Can you work these out from the model? Positions are in its coordinate system, mm. Coordinates: 2 decimals unless noted, no trailing zeros. Loops run counter-clockwise (first coordinate to the right, second up) from the corner with the lowest first, then second, coordinate; pieces in that order, holes last. Notation, with made-up numbers: M 86.5,-19.5 L 100.5,-19.5 A23 cw 100.5,1.5 Z; hole C 75,-29 d1. An arc over 180 degrees is marked long. Answer as a JSON object with one key per item and string values. Group by question number.
Item 1: Suppose I cut it at A-A (z = -2.5). Write out the boundary of the cut face in (x, y).
Item 2: I'm going to push flat-ended pins straight in: pin 1 Ø1.1 at (y, z) = (1.5, -24) entering from +X; pin 2 Ø1.5 at (x, z) = (1, 35.5) entering from -Y; pin 3 Ø0.7 at (y, z) = (1.5, -13) entering from -X; pin 4 Ø1.2 at (x, z) = (0, -3.5) entering from +Y. Where does each tip first touch, or does it pass through?
Item 3: Suppose I cut it at B-B (x = 0). Write out the boundary of the cut face in (y, z).
Item 4: Suppose I cut it at C-C (y = 1.6). Write out the boundary of the cut face in (x, z).
Item 5: If I drill on line 1 (Z direction, x = -0.05, y = 3.7); line 2 (Y direction, x = 1.05, z = -36); line 3 (X direction, y = 1.6, z = 16.5), over which ranges is the centre line in solid material (lowest first)?
```python
from build123d import *

# Parameters (mm, degrees)
SKETCH1_W           = 2.5
SKETCH1_H           = 105
BOSS_EXTRUDE1_DEPTH = 0.8
SKETCH2_W           = 1.9
SKETCH2_H           = 105
BOSS_EXTRUDE2_DEPTH = 1.4
SKETCH3_W           = 2.5
SKETCH3_H           = 105
BOSS_EXTRUDE3_DEPTH = 0.8
SKETCH4_R           = 0.65
BOSS_EXTRUDE4_DEPTH = 0.9


with BuildPart() as part:
    # Sketch1 → Boss-Extrude1 (new body)
    with BuildSketch(Plane(origin=(0, 0, 0), x_dir=(1, 0, 0), z_dir=(0, 1, 0))):
        Rectangle(SKETCH1_W, SKETCH1_H)
    extrude(amount=BOSS_EXTRUDE1_DEPTH)

    # Sketch2 → Boss-Extrude2 (add)
    with BuildSketch(Plane(origin=(0, 0.8, 0), x_dir=(1, 0, 0), z_dir=(0, 1, 0))):
        Rectangle(SKETCH2_W, SKETCH2_H)
    extrude(amount=BOSS_EXTRUDE2_DEPTH)

    # Sketch3 → Boss-Extrude3 (add)
    with BuildSketch(Plane(origin=(0, 2.2, 0), x_dir=(1, 0, 0), z_dir=(0, 1, 0))):
        Rectangle(SKETCH3_W, SKETCH3_H)
    extrude(amount=BOSS_EXTRUDE3_DEPTH)

    # Sketch4 → Boss-Extrude4 (add)
    with BuildSketch(Plane(origin=(0, 3, 0), x_dir=(1, 0, 0), z_dir=(0, 1, 0))):
        with Locations(Location((0, 18.75, 0), (0, 0, 270))):
            Circle(SKETCH4_R)
        with Locations(Location((0, -18.75, 0), (0, 0, 270))):
            Circle(SKETCH4_R)
        with Locations(Location((0, 48.75, 0), (0, 0, 270))):
            Circle(SKETCH4_R)
        with Locations(Location((0, -48.75, 0), (0, 0, 270))):
            Circle(SKETCH4_R)
    extrude(amount=BOSS_EXTRUDE4_DEPTH)


solid = part.part
```
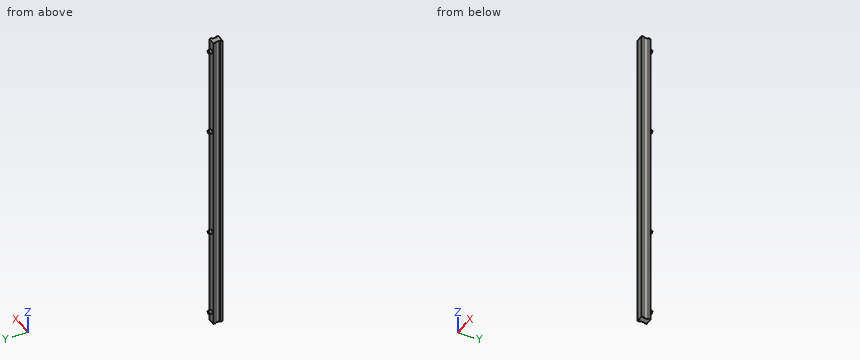
From the geometry:
{
 "1": {"outline": "M -1.25,0 L 1.25,0 L 1.25,0.8 L 0.95,0.8 L 0.95,2.2 L 1.25,2.2 L 1.25,3 L -1.25,3 L -1.25,2.2 L -0.95,2.2 L -0.95,0.8 L -1.25,0.8 Z"},
 "2": {"pin 1": "x = 0.95", "pin 2": "y = 0", "pin 3": "x = -0.95", "pin 4": "y = 3"},
 "3": {"outline": "M 0,-52.5 L 3,-52.5 L 3,-49.4 L 3.9,-49.4 L 3.9,-48.1 L 3,-48.1 L 3,-19.4 L 3.9,-19.4 L 3.9,-18.1 L 3,-18.1 L 3,18.1 L 3.9,18.1 L 3.9,19.4 L 3,19.4 L 3,48.1 L 3.9,48.1 L 3.9,49.4 L 3,49.4 L 3,52.5 L 0,52.5 Z"},
 "4": {"outline": "M -0.95,-52.5 L 0.95,-52.5 L 0.95,52.5 L -0.95,52.5 Z"},
 "5": {"line 1": "-49.4 to -48.1, -19.4 to -18.1, 18.1 to 19.4, 48.1 to 49.4", "line 2": "0 to 0.8, 2.2 to 3", "line 3": "-0.95 to 0.95"}
}
